from build123d import *

# Parameters (mm, degrees)
F0_W         = 55
F0_H         = 40
F1_DEPTH     = 0.8
F3_DEPTH     = 10
F2_R         = 3.75
F2_R_2       = 2.75
F4_DEPTH     = 8
F5_SIZE      = 0.5
F6_W         = 12.8945924119
F6_H         = 3
F7_DEPTH     = 1.5
F8_SIZE      = 1.49999
F9_SIZE      = 1.49999
F10_W        = 12.8768104754
F10_H        = 3
F11_DEPTH    = 1.5
F12_SIZE     = 1.49999
F13_W        = 12.9808257885
F13_H        = 3
F14_DEPTH    = 1.5
F15_SIZE     = 1.49999
F16_W        = 12.9808257885
F16_H        = 3
F17_DEPTH    = 1.5
F18_SIZE     = 1.49999
F19_T1_DEPTH = 59.8989794856
F19_T3_DEPTH = 44.8989794856


# Not quite as in the source:
# - a fillet or chamfer that OpenCascade refuses, or shapes differently, is made with other operations: its cross-section is extruded or revolved along the edge and cut away or added
# - a fillet or chamfer is up to 0.001 mm smaller than in the source, because OpenCascade refuses the exact size


with BuildPart() as f1:
    # F0 (on Top) → F1 (new body)
    with BuildSketch(Plane.XY):
        Rectangle(F0_W, F0_H)
    extrude(amount=F1_DEPTH)

    # F2 (on face) → F3 (join)
    with BuildSketch(Plane.XY.offset(0.8)):
        Polygon((7.1650690396, 12.9448085418), (8.2134181145, 14.8388137473), (-4.68486218, 16.3003894709), (-4.0868929955, 14.2198308067), align=None)
        with BuildLine():
            Line((-8.2134181145, -14.8388137473), (4.5991771643, -16.2906800263))
            ThreePointArc((4.5991771643, -16.2906800263), (4.6374749925, -16.2797221091), (4.6757470388, -16.268674482))
            Line((4.6757470388, -16.268674482), (4.0868929955, -14.2198308067))
            Line((4.0868929955, -14.2198308067), (-7.1650690396, -12.9448085418))
            Line((-7.1650690396, -12.9448085418), (-8.2134181145, -14.8388137473))
        make_face()
        Polygon((-14.8388137473, 8.2134181145), (-16.3003894709, -4.68486218), (-14.2198308067, -4.0868929955), (-12.9448085418, 7.1650690396), align=None)
        with BuildLine():
            Line((14.8505253486, -8.1100642381), (16.3003894709, 4.68486218))
            Line((16.3003894709, 4.68486218), (14.2198308067, 4.0868929955))
            Line((14.2198308067, 4.0868929955), (12.9448085418, -7.1650690396))
            Line((12.9448085418, -7.1650690396), (14.8041096105, -8.1942090597))
            ThreePointArc((14.8041096105, -8.1942090597), (14.8273769365, -8.1521694464), (14.8505253486, -8.1100642381))
        make_face()
    extrude(amount=F3_DEPTH)

    # F2 (on face) → F4 (join)
    with BuildSketch(Plane.XY.offset(0.8)):
        with Locations((22.4918836008, 10.0589259832)):
            Circle(F2_R)
        with Locations((22.4918836008, 10.0589259832)):
            Circle(F2_R_2, mode=Mode.SUBTRACT)
        with Locations((-22.6081163992, 10.0589259832)):
            Circle(F2_R)
        with Locations((-22.6081163992, 10.0589259832)):
            Circle(F2_R_2, mode=Mode.SUBTRACT)
    extrude(amount=F4_DEPTH)

    # F5
    f5_edges = [f1.edges().sort_by_distance(p)[0] for p in [
        (-26.358116, 10.058926, 8.8),
        (18.741884, 10.058926, 8.8),
    ]]
    chamfer(f5_edges, length=F5_SIZE)

    # F6 (on face) → F7 (join)
    with BuildSketch(Plane(origin=(-1.7642779672, -15.5696016091, 0), x_dir=(0.9936409674, -0.1125949726, 0), z_dir=(-0.1125949726, -0.9936409674, 0))):
        with Locations((-0.0431166883, 9.3)):
            Rectangle(F6_W, F6_H)
    extrude(amount=F7_DEPTH)

    # F8 (size 1.5 in the source; OpenCascade refuses exactly that, so slightly less here)
    f8_edges = [f1.edges().sort_by_distance(p)[0] for p in [
        (-1.976013, -17.055208, 7.8),
    ]]
    chamfer(f8_edges, length=F8_SIZE)

    # F9 (size 1.5 in the source; OpenCascade refuses exactly that, so slightly less here)
    f9_edges = [f1.edges().sort_by_distance(p)[0] for p in [
        (-8.382311, -16.329275, 10.049995),
        (4.430285, -17.781141, 10.049995),
    ]]
    chamfer(f9_edges, length=F9_SIZE)

    # F10 (on face) → F11 (join)
    with BuildSketch(Plane(origin=(15.5696016091, -1.7642779672, 0), x_dir=(0.1125949726, 0.9936409674, 0), z_dir=(0.9936409674, -0.1125949726, 0))):
        with Locations((0.0520076565, 9.3)):
            Rectangle(F10_W, F10_H)
    extrude(amount=F11_DEPTH)

    # F12 (size 1.5 in the source; OpenCascade refuses exactly that, so slightly less here)
    f12_edges = [f1.edges().sort_by_distance(p)[0] for p in [
        (17.065919, -1.881493, 7.8),
        (16.340987, -8.278957, 9.3),
        (17.790851, 4.51597, 9.3),
    ]]
    chamfer(f12_edges, length=F12_SIZE)

    # F13 (on face) → F14 (join)
    with BuildSketch(Plane(origin=(1.7642779672, 15.5696016091, 0), x_dir=(-0.9936409674, 0.1125949726, 0), z_dir=(0.1125949726, 0.9936409674, 0))):
        with Locations((0, 9.3)):
            Rectangle(F13_W, F13_H)
    extrude(amount=F14_DEPTH)

    # F15 (size 1.5 in the source; OpenCascade refuses exactly that, so slightly less here)
    f15_edges = [f1.edges().sort_by_distance(p)[0] for p in [
        (8.382311, 16.329275, 9.3),
        (1.93317, 17.060063, 7.8),
        (-4.51597, 17.790851, 9.3),
    ]]
    chamfer(f15_edges, length=F15_SIZE)

    # F16 (on face) → F17 (join)
    with BuildSketch(Plane(origin=(-15.5696016091, 1.7642779672, 0), x_dir=(-0.1125949726, -0.9936409674, 0), z_dir=(-0.9936409674, 0.1125949726, 0))):
        with Locations((0, 9.3)):
            Rectangle(F16_W, F16_H)
    extrude(amount=F17_DEPTH)

    # F18 (size 1.5 in the source; OpenCascade refuses exactly that, so slightly less here)
    f18_edges = [f1.edges().sort_by_distance(p)[0] for p in [
        (-16.329275, 8.382311, 9.3),
        (-17.060063, 1.93317, 7.8),
        (-17.790851, -4.51597, 9.3),
    ]]
    chamfer(f18_edges, length=F18_SIZE)

    # F19: fillet of radius 1 on 4 edges, made by hand

    # F19_s2 → F19_t1 (cut)
    with BuildSketch(Plane.YZ.offset(-29.9494897428)):
        with BuildLine():
            ThreePointArc((-20, 0.8), (-19.6526596349, 0.2254033308), (-19.0202041029, 0))
            Line((-19.0202041029, 0), (-20, 0))
            Line((-20, 0), (-20, 0.8))
        make_face()
        with BuildLine():
            ThreePointArc((20, 0.8), (19.6526596349, 0.2254033308), (19.0202041029, 0))
            Line((19.0202041029, 0), (20, 0))
            Line((20, 0), (20, 0.8))
        make_face()
    extrude(amount=F19_T1_DEPTH, mode=Mode.SUBTRACT)

    # F19_s4 → F19_t3 (cut)
    with BuildSketch(Plane.XZ.offset(-22.4494897428)):
        with BuildLine():
            ThreePointArc((27.5, 0.8), (27.1526596349, 0.2254033308), (26.5202041029, 0))
            Line((26.5202041029, 0), (27.5, 0))
            Line((27.5, 0), (27.5, 0.8))
        make_face()
        with BuildLine():
            ThreePointArc((-27.5, 0.8), (-27.1526596349, 0.2254033308), (-26.5202041029, 0))
            Line((-26.5202041029, 0), (-27.5, 0))
            Line((-27.5, 0), (-27.5, 0.8))
        make_face()
    extrude(amount=F19_T3_DEPTH, mode=Mode.SUBTRACT)


solid = f1.part
Source: CAD feature listing. Evaluate the final solid. Frame: model axes, mm. A direction names the side the tool comes from. Coordinates: 2 decimals unless noted, no trailing zeros. Write each loop counter-clockwise with the first axis right and the second up, starting at its lowest first coordinate (ties: lowest second). Pieces come first, ordered by that corner, then holes. Notation, with made-up numbers: M 0,87.5 L 53,87.5 A36 cw 53,126.5 Z; hole C -25,-9 d11. An arc over 180 degrees is marked long. Use a Markdown table: item, result.
1) Mould query, pull axis Z, two halves, no side actions, for faces 1 (the flat face through (15, -2, 10.8)), 2 (the flat face through (15.27, 4.39, 5.73)), 3 (the flat face through (-16.315, 1.94, 8.56)). Classes: pulls with the +Z half, pulls with the -Z half, needs draft (parallel to the pull), parting line crosses it, or undercut.
Conclusion:
| item | result |
|---|---|
| face 1 | pulls with the +Z half |
| face 2 | needs draft |
| face 3 | undercut |
2) First-contact query: pin 1 Ø5 at (x, z) = (-12.5, 5.5) entering from -Y; pin 2 Ø1.6 at (x, y) = (-23, 11) entering from +Z; pin 3 Ø5 at (y, z) = (2.5, 5.5) entering from +X. Flat tips, straight axial feed; report the tip coordinate or a pass-through.
Conclusion:
| item | result |
|---|---|
| pin 1 | stops at y = -4.31 |
| pin 2 | stops at z = 0.8 |
| pin 3 | stops at x = 16.3 |
3) Section C-C, the plane x = 9.5. Output: boundary loops of the cut face in (y, z), then the cut area to 3 significant figures.
Conclusion:
| item | result |
|---|---|
| outline | M -20,0.8 A1 ccw -19.02,0 L 19.02,0 A1 ccw 20,0.8 Z |
| area | 31.6 mm^2 |
4) Ray query, L1, parallel to X at y = 9, z = 6; L2, parallel to Z at x = 21, y = 4.5; L3, parallel to Y at x = -3, z = 7.5. Return the intervals inside material, ascending.
Conclusion:
| item | result |
|---|---|
| L1 | x = -26.21 to -25.15, -20.07 to -19.01, 18.89 to 19.95, 25.03 to 26.09 |
| L2 | z = 0 to 0.8 |
| L3 | y = -15.43 to -13.42, 14.1 to 16.11 |
5) Section A-A, the plane z = 4.5. Output: boundary loops of the cut face in (x, y), then the cut area to 3 significant figures.
Conclusion:
| item | result |
|---|---|
| outline | C -22.61,10.06 d7.5; M -16.3,-4.68 L -14.22,-4.09 L -12.94,7.17 L -14.84,8.21 Z; M -8.21,-14.84 L 4.6,-16.29 A17 ccw 4.68,-16.27 L 4.09,-14.22 L -7.17,-12.94 Z; M -4.68,16.3 L -4.09,14.22 L 7.17,12.94 L 8.21,14.84 Z; M 12.94,-7.17 L 14.8,-8.19 A17 ccw 14.85,-8.11 L 16.3,4.68 L 14.22,4.09 Z; C 22.49,10.06 d7.5; hole C -22.61,10.06 d5.5; hole C 22.49,10.06 d5.5 |
| area | 138 mm^2 |
6) Reachability of faces 4 (the flat face through (-7.543, -15.68, 9.612)), 5 (the flat face through (22, 10, 0.8)), 6 (the flat face through (23, 13, 8.8)) from +Z, -Z, +X, -X, +Y, -Y: full face, straight path, thin tool, end or side. Return the list, or none.
Conclusion:
| item | result |
|---|---|
| face 4 | +Z, -X, -Y |
| face 5 | +Z |
| face 6 | +Z, +X, +Y, -Y |
